The model under review builds one solid part; all positions refer to its coordinate system, in mm. A direction names the side the tool comes from. Give positions to 0.01 mm unless a question says otherwise; leave off trailing zeros. Order: outer loops, then holes, each group sorted by start corner. A loop starts at its lowest first (then second) coordinate and runs counter-clockwise, first axis right, second up. Notation, with made-up numbers: (79, 51.25) - (103, 51.25) arc R20 ccw to (103, 56.25) - close; hole circle Ø5 at (61, -30). An arc over 180 degrees is marked (long way). Put each result on its own line as item: value.
```python
from build123d import *

# Parameters (mm, degrees)
F0_W     = 80
F0_H     = 80
F1_DEPTH = 40
F3_DEPTH = 40.001
F4_R     = 4
F5_DEPTH = 40.001
F6_R     = 8
F7_DEPTH = 1


with BuildPart() as f1:
    # F0 (on Right) → F1 (new body)
    with BuildSketch(Plane.YZ):
        Rectangle(F0_W, F0_H)
    extrude(amount=F1_DEPTH)

    # F2 (on face) → F3 (cut, through all)
    with BuildSketch(Plane.YZ.offset(40)):
        with BuildLine():
            ThreePointArc((-40, 32), (-36.221541, 36.221541), (-32, 40))
            Line((-32, 40), (-40, 40))
            Line((-40, 40), (-40, 32))
        make_face()
        with BuildLine():
            ThreePointArc((-32, -40), (-36.221541, -36.221541), (-40, -32))
            Line((-40, -32), (-40, -40))
            Line((-40, -40), (-32, -40))
        make_face()
        with BuildLine():
            ThreePointArc((40, -32), (36.221541, -36.221541), (32, -40))
            Line((32, -40), (40, -40))
            Line((40, -40), (40, -32))
        make_face()
        with BuildLine():
            ThreePointArc((32, 40), (36.221541, 36.221541), (40, 32))
            Line((40, 32), (40, 40))
            Line((40, 40), (32, 40))
        make_face()
    extrude(amount=-F3_DEPTH, mode=Mode.SUBTRACT)

    # F4 (on face) → F5 (cut, through all)
    with BuildSketch(Plane(origin=(0, 0, 0), x_dir=(0, -1, 0), z_dir=(-1, 0, 0))):
        Circle(F4_R)
    extrude(amount=-F5_DEPTH, mode=Mode.SUBTRACT)

    # F6 (on face) → F7 (join)
    with BuildSketch(Plane(origin=(0, 0, 0), x_dir=(0, -1, 0), z_dir=(-1, 0, 0))):
        with Locations((26.162951, 26.162951)):
            Circle(F6_R)
    extrude(amount=F7_DEPTH)


solid = f1.part
```
(1) Take a section at A-A, the plane y = 0. Write out the cut boundary in (x, z), then the cut area to 3 significant figures.
The answers:
outline: (0, -40) - (40, -40) - (40, -4) - (0, -4) - close; (0, 4) - (40, 4) - (40, 40) - (0, 40) - close
area: 2,880 mm^2
(2) The part is to be moulded in two halves that separate along Z. For faces 1 (the cylindrical face through (19.72, 0.867, -3.905)), 2 (the cylindrical face through (20.28, 36.278, -36.165)), 3 (the flat face through (-1, -26, 26)), 4 (the cylindrical face through (20.28, -36.278, 36.165)), say which applies: pulls with the +Z half, pulls with the -Z half, needs draft (parallel to the pull), parting line crosses it, or undercut.
The answers:
face 1: undercut
face 2: pulls with the -Z half
face 3: needs draft
face 4: pulls with the +Z half
(3) For faces 5 (the cylindrical face through (20.28, -36.165, -36.278)), 6 (the cylindrical face through (-0.493, -33.553, 23.099)), list the 3-axis set-ups (+Z, -Z, +X, -X, +Y, -Y) from which the entire face can be reached by the end or side of a thin tool; tool diameter is ignored.
The answers:
face 5: -Z, +X, -X, -Y
face 6: -X
(4) Take a section at C-C, the plane x = 29.5. Write out the cut boundary in (y, z).
The answers:
outline: (-40, -32) arc R51.22 ccw to (-32, -40) - (32, -40) arc R51.22 ccw to (40, -32) - (40, 32) arc R51.22 ccw to (32, 40) - (-32, 40) arc R51.22 ccw to (-40, 32) - close; hole circle Ø8 at (0, 0)
(5) Clearance check with a flat-ended pin moving along its axis: pin 1 Ø12 at (y, z) = (20, -22.5) entering from -X. State where the tip first meets the part, or that it passes through.
The answers:
pin 1: x = 0
(6) Wall thickness on L1, parallel to Z at x = 22.5, y = 0; L2, parallel to X at y = -16, z = 11; L3, parallel to Z at x = 5.5, y = 3.5: over which ranges is each line inside the solid? List them lowest first.
The answers:
L1: -40 to -4, 4 to 40
L2: 0 to 40
L3: -40 to -1.94, 1.94 to 40
(7) Take a section at D-D, the plane y = -20. Write out the cut boundary in (x, z), then the cut area to 3 significant figures.
The answers:
outline: (-1, 21.06) - (0, 21.06) - (0, -40) - (40, -40) - (40, 40) - (0, 40) - (0, 31.26) - (-1, 31.26) - close
area: 3,210 mm^2
